Check sheet for the drawn part. Datum: minimum x, y, z corner. Units: mm. A direction names the side the tool comes from. Coordinates: 2 decimals unless noted, no trailing zeros. Write each loop counter-clockwise with the first axis right and the second up, starting at its lowest first coordinate (ties: lowest second). Pieces come first, ordered by that corner, then holes. Notation, with made-up numbers: (44, -26) - (68, -26) arc R27 cw to (68, 4) - close; hole circle Ø7 at (84.25, -25). An arc over 180 degrees is marked (long way). Use one line per item in the form item = value. Start each with the question number.
1. Cross-section at C-C on y = 60. Record the boundary of the cut face in (x, z).
2. Cross-section at B-B on y = 33. Record the boundary of the cut face in (x, z).
3. Scan lines: line 1 along Z through (x, y) = (47, 17); line 2 along X through (y, z) = (38, 6); line 3 along X through (y, z) = (19.5, 4.5). Record each from-to range of solid material in increasing order.
4. Cross-section at A-A on z = 6.75. Record the boundary of the cut face in (x, y).
5. Cross-section at D-D on x = 77.5. Record the boundary of the cut face in (y, z).
6. Tool access check on the marked faces 1 and 2. Record the directions out of +Z, -Z, +X, -X, +Y, -Y that give a thin tool (end or side, any length) a straight path to the whole face; none if there is none.
7. Go/stop test with flat-tipped pins: pin 1 Ø4 at (y, z) = (35, 8) entering from -X; pin 2 Ø5 at (y, z) = (14, 7) entering from +X; pin 3 Ø4.5 at (x, z) = (112.5, 5.5) entering from +Y. Record where each tip stops, or that it passes through.
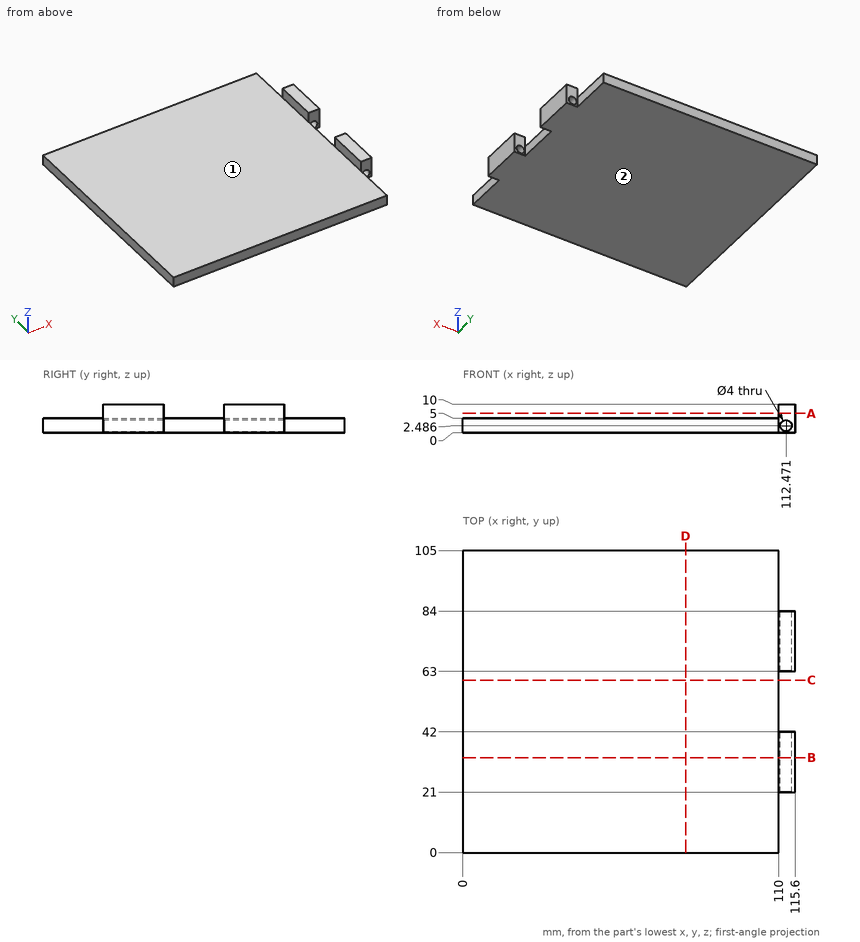
Final values:
q1.outline = (0, 0) - (110, 0) - (110, 5) - (0, 5) - close
q2.outline = (0, 0) - (115.6, 0) - (115.6, 10) - (110, 10) - (110, 5) - (0, 5) - close; hole circle Ø4 at (112.47, 2.49)
q3.line_1 = 0 to 5
q3.line_2 = 110 to 115.6
q3.line_3 = 0 to 110
q4.outline = (110, 21) - (115.6, 21) - (115.6, 42) - (110, 42) - close; (110, 63) - (115.6, 63) - (115.6, 84) - (110, 84) - close
q5.outline = (0, 0) - (105, 0) - (105, 5) - (0, 5) - close
q6.face_1 = +Z, -X, +Y, -Y
q6.face_2 = -Z, +X, -X, +Y, -Y
q7.pin_1 = 110
q7.pin_2 = 110
q7.pin_3 = 84
